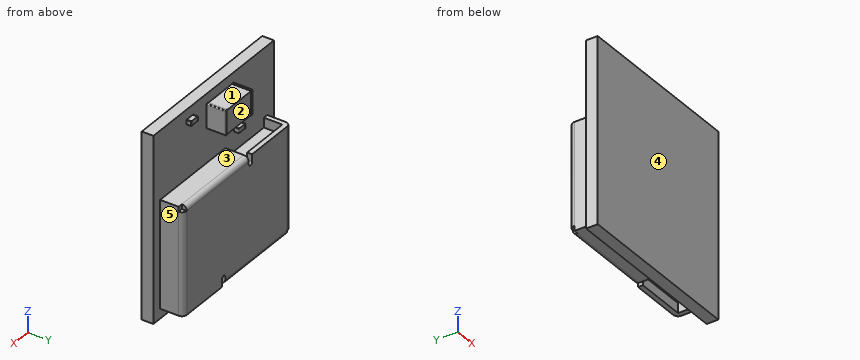
from build123d import *

# Parameters (mm, degrees)
SKETCH1_W           = 9
SKETCH1_H           = 9.5
BOSS_EXTRUDE1_DEPTH = 0.6
SKETCH2_W           = 8
SKETCH2_H           = 5.5
BOSS_EXTRUDE2_DEPTH = 1.2
CUT_EXTRUDE1_DEPTH  = 1.2
SKETCH4_W           = 0.25
SKETCH4_H           = 0.25
CUT_EXTRUDE2_DEPTH  = 0.25
FILLET1_R           = 0.25
SKETCH5_W           = 2.875
SKETCH5_H           = 0.95
CUT_EXTRUDE3_DEPTH  = 0.5
SKETCH7_W           = 2.875
SKETCH7_H           = 0.95
CUT_EXTRUDE4_DEPTH  = 0.5
BOSS_EXTRUDE3_DEPTH = 1
SKETCH9_W           = 1.778
SKETCH9_H           = 1.2192
CUT_EXTRUDE5_DEPTH  = 0.0254
FILLET2_R           = 0.0508
BOSS_EXTRUDE4_DEPTH = 0.254
SKETCH11_W          = 0.4318
SKETCH11_H          = 0.2286
CUT_EXTRUDE6_DEPTH  = 0.0127
FILLET3_R           = 0.0254


with BuildPart() as part:
    # Sketch1 → Boss-Extrude1 (new body)
    with BuildSketch(Plane(origin=(0, 0, 0), x_dir=(1, 0, 0), z_dir=(0, 1, 0))):
        Rectangle(SKETCH1_W, SKETCH1_H)
    extrude(amount=BOSS_EXTRUDE1_DEPTH)

    # Sketch2 → Boss-Extrude2 (add)
    with BuildSketch(Plane(origin=(0, 0.6, 0), x_dir=(1, 0, 0), z_dir=(0, 1, 0))):
        with Locations((0, 1.5)):
            Rectangle(SKETCH2_W, SKETCH2_H)
    extrude(amount=BOSS_EXTRUDE2_DEPTH)

    # Sketch3 → Cut-Extrude1 (cut)
    with BuildSketch(Plane(origin=(0, 1.8, 0), x_dir=(1, 0, 0), z_dir=(0, 1, 0))):
        with BuildLine():
            Line((0.875, 4.25), (0.875, 3.875))
            ThreePointArc((0.875, 3.875), (1, 3.75), (1.125, 3.875))
            Line((1.125, 3.875), (1.125, 4.25))
            Line((1.125, 4.25), (0.875, 4.25))
        make_face()
        with BuildLine():
            Line((-1.125, -0.875), (-1.125, -1.25))
            Line((-1.125, -1.25), (-0.875, -1.25))
            Line((-0.875, -1.25), (-0.875, -0.875))
            ThreePointArc((-0.875, -0.875), (-1, -0.75), (-1.125, -0.875))
        make_face()
    extrude(amount=-CUT_EXTRUDE1_DEPTH, mode=Mode.SUBTRACT)

    # Sketch4 → Cut-Extrude2 (cut)
    with BuildSketch(Plane(origin=(0, 1.8, 0), x_dir=(1, 0, 0), z_dir=(0, 1, 0))):
        with Locations((3.875, -1.125)):
            Rectangle(SKETCH4_W, SKETCH4_H)
        with Locations((-3.875, 4.125)):
            Rectangle(SKETCH4_W, SKETCH4_H)
    extrude(amount=-CUT_EXTRUDE2_DEPTH, mode=Mode.SUBTRACT)

    # Fillet1
    fillet1_edges = [part.edges().sort_by_distance(p)[0] for p in [
        (-1.4375, 1.8, -4.25),
        (4, 1.8, -1.625),
        (1.4375, 1.8, 1.25),
        (-4, 1.8, -1.375),
    ]]
    fillet(fillet1_edges, radius=FILLET1_R)

    # Sketch5 → Cut-Extrude3 (cut)
    with BuildSketch(Plane.XY.offset(1.25)):
        with Locations((-2.3125, 1.075)):
            Rectangle(SKETCH5_W, SKETCH5_H)
    extrude(amount=-CUT_EXTRUDE3_DEPTH, mode=Mode.SUBTRACT)

    # Sketch7 → Cut-Extrude4 (cut)
    with BuildSketch(Plane(origin=(0, 0, -4.25), x_dir=(-1, 0, 0), z_dir=(0, 0, -1))):
        with Locations((-2.3125, 1.075)):
            Rectangle(SKETCH7_W, SKETCH7_H)
    extrude(amount=-CUT_EXTRUDE4_DEPTH, mode=Mode.SUBTRACT)

    # Sketch8 → Boss-Extrude3 (add)
    with BuildSketch(Plane(origin=(0, 0.6, 0), x_dir=(1, 0, 0), z_dir=(0, 1, 0))):
        Polygon((-1.5, -2.98), (-1.373, -2.98), (-1.373, -3.0054), (0.405, -3.0054), (0.405, -2.98), (0.532, -2.98), (0.532, -4.25), (0.405, -4.25), (0.405, -4.2246), (-1.373, -4.2246), (-1.373, -4.25), (-1.5, -4.25), align=None)
    extrude(amount=BOSS_EXTRUDE3_DEPTH)

    # Sketch9 → Cut-Extrude5 (cut)
    with BuildSketch(Plane(origin=(0, 1.6, 0), x_dir=(1, 0, 0), z_dir=(0, 1, 0))):
        with Locations((-0.484, -3.615)):
            Rectangle(SKETCH9_W, SKETCH9_H)
    extrude(amount=-CUT_EXTRUDE5_DEPTH, mode=Mode.SUBTRACT)

    # Fillet2
    fillet2_edges = [part.edges().sort_by_distance(p)[0] for p in [
        (-1.5, 1.1, 2.98),
        (-1.5, 1.1, 4.25),
        (0.532, 1.1, 4.25),
        (0.532, 1.1, 2.98),
        (-1.5, 1.6, 3.615),
        (-1.4365, 1.6, 4.25),
        (0.4685, 1.6, 4.25),
        (0.532, 1.6, 3.615),
        (0.4685, 1.6, 2.98),
        (-1.4365, 1.6, 2.98),
    ]]
    fillet(fillet2_edges, radius=FILLET2_R)

    # Sketch10 → Boss-Extrude4 (add)
    with BuildSketch(Plane(origin=(0, 0.6, 0), x_dir=(1, 0, 0), z_dir=(0, 1, 0))):
        Polygon((-2.033, -1.726), (-1.9949, -1.726), (-1.9949, -1.7387), (-1.5631, -1.7387), (-1.5631, -1.726), (-1.525, -1.726), (-1.525, -1.98), (-1.5631, -1.98), (-1.5631, -1.9673), (-1.9949, -1.9673), (-1.9949, -1.98), (-2.033, -1.98), align=None)
        Polygon((1.532, -3.996), (1.5701, -3.996), (1.5701, -4.0087), (2.0019, -4.0087), (2.0019, -3.996), (2.04, -3.996), (2.04, -4.25), (2.0019, -4.25), (2.0019, -4.2373), (1.5701, -4.2373), (1.5701, -4.25), (1.532, -4.25), align=None)
    extrude(amount=BOSS_EXTRUDE4_DEPTH)

    # Sketch11 → Cut-Extrude6 (cut)
    with BuildSketch(Plane(origin=(0, 0.854, 0), x_dir=(1, 0, 0), z_dir=(0, 1, 0))):
        with Locations((-1.779, -1.853)):
            Rectangle(SKETCH11_W, SKETCH11_H)
        with Locations((1.786, -4.123)):
            Rectangle(SKETCH11_W, SKETCH11_H)
    extrude(amount=-CUT_EXTRUDE6_DEPTH, mode=Mode.SUBTRACT)

    # Fillet3
    fillet3_edges = [part.edges().sort_by_distance(p)[0] for p in [
        (-2.033, 0.727, 1.726),
        (-2.033, 0.727, 1.98),
        (-1.525, 0.727, 1.98),
        (-1.525, 0.727, 1.726),
        (-2.033, 0.854, 1.853),
        (-2.01395, 0.854, 1.98),
        (-1.54405, 0.854, 1.98),
        (-1.525, 0.854, 1.853),
        (-1.54405, 0.854, 1.726),
        (-2.01395, 0.854, 1.726),
        (1.532, 0.727, 3.996),
        (1.532, 0.727, 4.25),
        (2.04, 0.727, 4.25),
        (2.04, 0.727, 3.996),
        (1.532, 0.854, 4.123),
        (1.55105, 0.854, 4.25),
        (2.02095, 0.854, 4.25),
        (2.04, 0.854, 4.123),
        (2.02095, 0.854, 3.996),
        (1.55105, 0.854, 3.996),
    ]]
    fillet(fillet3_edges, radius=FILLET3_R)


solid = part.part
The model under review builds one solid part; all positions refer to its coordinate system, in mm. Face numbers are marked on the shaded views. A direction names the side the tool comes from. Coordinates: 2 decimals unless noted, no trailing zeros. Loops run counter-clockwise (first coordinate to the right, second up) from the corner with the lowest first, then second, coordinate; pieces in that order, holes last. Notation, with made-up numbers: (5, -30.5) -> (22, -30.5) arc R31 cw to (22, -3.5) -> close; hole circle Ø8 at (-3, 64). An arc over 180 degrees is marked (long way). Use a Markdown table: item, result. Add a question column.
1. Clearance check with flat-ended pins moving along their axes: pin 1 Ø0.5 at (x, y) = (0, 1) entering from -Z; pin 2 Ø0.5 at (y, z) = (1, 3.5) entering from +X; pin 3 Ø0.5 at (x, y) = (2.5, 1) entering from +Z; pin 4 Ø3 at (x, z) = (3, -0.5) entering from -Y. State where each tip first meets the part, or that it passes through.
2. Add section C-C on z = 3.25. Write out the cut boundary in (x, y) (3 decimals).
3. Draft analysis for pull direction Z (two halves, no side actions). For the marked faces 1, 2 and 3, state which applies: pulls with the +Z half, pulls with the -Z half, needs draft (parallel to the pull), parting line crosses it, or undercut.
4. To check wall thickness, follow line 1 (Z direction, x = 0.75, y = 1.1); line 2 (Z direction, x = 0, y = 0.95); line 3 (X direction, y = 0.7, z = -1.5). State the ranges of each line that lie inside material, in increasing order.
5. Add section D-D on x = 2.75. Write out the cut boundary in (y, z), plus the area to 3 significant figures.
6. Add section A-A on y = 1.05. Write out the cut boundary in (x, z) (3 decimals).
7. Machinability: for the marked faces 4 and 5, which of the approach directions +Z, -Z, +X, -X, +Y, -Y give a long, thin tool a straight path to every point of the face, cutting with its end or side? Answer none if there is none.
8. Add section B-B on x = -0.5. Write out the cut boundary in (y, z).
Returned:
| question | item | result |
|---|---|---|
| 1 | pin 1 | stops at z = -4.25 |
| 1 | pin 2 | stops at x = 0.53 |
| 1 | pin 3 | stops at z = 1.25 |
| 1 | pin 4 | stops at y = 0 |
| 2 | outline | (-4.5, 0) -> (4.5, 0) -> (4.5, 0.6) -> (0.532, 0.6) -> (0.532, 1.549) arc R0.051 ccw to (0.481, 1.6) -> (0.405, 1.6) -> (0.405, 1.575) -> (-1.373, 1.575) -> (-1.373, 1.6) -> (-1.449, 1.6) arc R0.051 ccw to (-1.5, 1.549) -> (-1.5, 0.6) -> (-4.5, 0.6) -> close |
| 3 | face 1 | pulls with the +Z half |
| 3 | face 2 | needs draft |
| 3 | face 3 | undercut |
| 4 | line 1 | z = -4.25 to 1.25 |
| 4 | line 2 | z = -4.25 to 1.25, 3.01 to 4.22 |
| 4 | line 3 | x = -4 to 4 |
| 5 | outline | (0, -4.75) -> (0.6, -4.75) -> (0.6, -3.75) -> (1.55, -3.75) -> (1.55, -4.25) -> (1.8, -4.25) -> (1.8, 1) arc R0.25 ccw to (1.55, 1.25) -> (0.6, 1.25) -> (0.6, 4.75) -> (0, 4.75) -> close |
| 5 | area | 11.8 mm² |
| 6 | outline | (-4, -4.25) -> (0.875, -4.25) -> (0.875, -3.75) -> (3.75, -3.75) -> (3.75, -4.25) -> (4, -4.25) -> (4, 1.25) -> (-0.875, 1.25) -> (-0.875, 0.75) -> (-3.75, 0.75) -> (-3.75, 1.25) -> (-4, 1.25) -> close; (-1.5, 3.031) arc R0.051 ccw to (-1.449, 2.98) -> (-1.373, 2.98) -> (-1.373, 3.005) -> (0.405, 3.005) -> (0.405, 2.98) -> (0.481, 2.98) arc R0.051 ccw to (0.532, 3.031) -> (0.532, 4.199) arc R0.051 ccw to (0.481, 4.25) -> (0.405, 4.25) -> (0.405, 4.225) -> (-1.373, 4.225) -> (-1.373, 4.25) -> (-1.449, 4.25) arc R0.051 ccw to (-1.5, 4.199) -> close |
| 7 | face 4 | +Z, -Z, +X, -X, -Y |
| 7 | face 5 | +Z, -Z, +X, +Y |
| 8 | outline | (0, -4.75) -> (0.6, -4.75) -> (0.6, -4.25) -> (1.55, -4.25) arc R0.25 ccw to (1.8, -4) -> (1.8, 1) arc R0.25 ccw to (1.55, 1.25) -> (0.6, 1.25) -> (0.6, 3.01) -> (1.57, 3.01) -> (1.57, 4.22) -> (0.6, 4.22) -> (0.6, 4.75) -> (0, 4.75) -> close |
